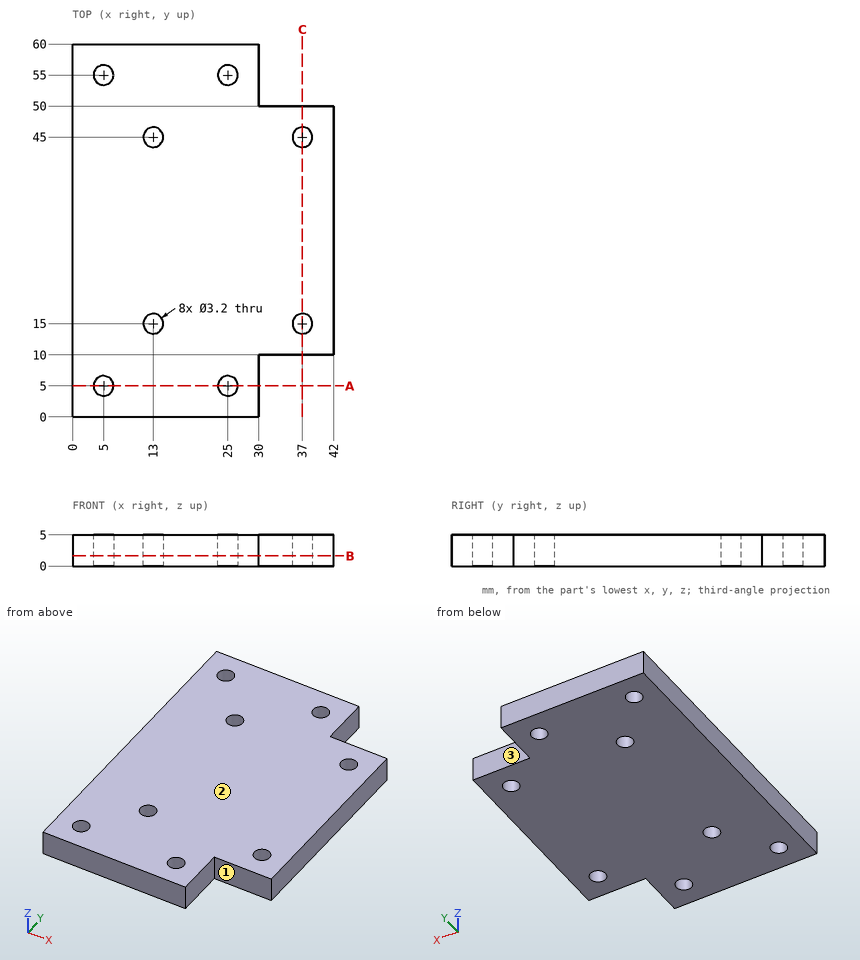
Source: three-view drawing plus pictorial views. Frame: mm from the lowest corner of the part. A direction names the side the tool comes from. Round coordinates to 2 decimals unless told otherwise and drop trailing zeros. Loops run counter-clockwise (first coordinate to the right, second up) from the corner with the lowest first, then second, coordinate; pieces in that order, holes last.
Item 1: Contact query for flat-ended pins moving along their axis: P1, Ø2.5, axis at x = 37, y = 15, coming from the +Z side; P2, Ø1, axis at x = 37, z = 4.5, coming from the +Y side. Output: stop coordinate, or through.
Checked values:
P1: passes through
P2: stops at y = 50
Item 2: Reachability of the marked faces 1, 2 and 3 from +Z, -Z, +X, -X, +Y, -Y: full face, straight path, thin tool, end or side. Return the list, or none.
Checked values:
face 1: +Z, -Z, +X, -Y
face 2: +Z, +X, -X, +Y, -Y
face 3: +Z, -Z, +X, +Y
Item 3: Line query: L1, parallel to Y at x = 5, z = 1.3; L2, parallel to Y at x = 37, z = 2.6; L3, parallel to X at y = 55, z = 1.5. Output: solid intervals per line, ascending.
Checked values:
L1: y = 0 to 3.4, 6.6 to 53.4, 56.6 to 60
L2: y = 10 to 13.4, 16.6 to 43.4, 46.6 to 50
L3: x = 0 to 3.4, 6.6 to 23.4, 26.6 to 30
Item 4: Section A-A, the plane y = 5. Output: boundary loops of the cut face in (x, z).
Checked values:
outline: (0, 0) - (3.4, 0) - (3.4, 5) - (0, 5) - close; (6.6, 0) - (23.4, 0) - (23.4, 5) - (6.6, 5) - close; (26.6, 0) - (30, 0) - (30, 5) - (26.6, 5) - close
Item 5: Section C-C, the plane x = 37. Output: boundary loops of the cut face in (y, z), plus the area to 3 significant figures.
Checked values:
outline: (10, 0) - (13.4, 0) - (13.4, 5) - (10, 5) - close; (16.6, 0) - (43.4, 0) - (43.4, 5) - (16.6, 5) - close; (46.6, 0) - (50, 0) - (50, 5) - (46.6, 5) - close
area: 168 mm2
Item 6: Section B-B, the plane z = 1.65. State how many separate pieces and enclosed holes the cut face has, plus the area to 3 significant figures.
Checked values:
separate pieces: 1
enclosed holes: 8
area: 2,220 mm2
